The model under review builds one solid part; all positions refer to its coordinate system, in mm. Face numbers are marked on the shaded views. A direction names the side the tool comes from. Round coordinates to 2 decimals unless told otherwise and drop trailing zeros. Order: outer loops, then holes, each group sorted by start corner. A loop starts at its lowest first (then second) coordinate and runs counter-clockwise, first axis right, second up.
1) Consider section C-C (z = 13). Give the boundary of the cut face in (x, y), then the cut area to 3 significant figures.
2) Consider section A-A (y = -25.5). Give the boundary of the cut face in (x, z), then the cut area to 3 significant figures.
3) Clearance check with flat-ended pins moving along their axes: P1, Ø1.5, axis at x = 12.5, z = 12.5, coming from the -Y side; P2, Ø5, axis at x = -13, z = 13, coming from the -Y side; P3, Ø10.5, axis at x = -5, z = 8, coming from the -Y side. State where each tip first meets the part, or that it passes through.
4) Machinability: for the marked faces 1 and 2, which of the approach directions +Z, -Z, +X, -X, +Y, -Y give a long, thin tool a straight path to every point of the face, cutting with its end or side? Answer none if there is none.
5) To check wall thickness, follow L1, parallel to Z at x = -13, y = -13.5; L2, parallel to Z at x = 14, y = -8; L3, parallel to Y at x = 13.5, z = -4.5. State the ranges of each line that lie inside material, in increasing order.
6) Consider section D-D (z = -4). Give the boundary of the cut face in (x, y), then the cut area to 3 significant figures.
7) Consider section B-B (x = 13). Give the boundary of the cut face in (y, z), then the cut area to 3 significant figures.
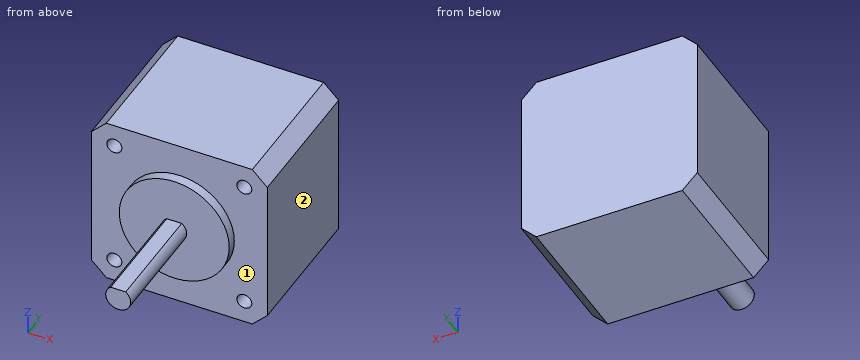
from build123d import *

# Parameters (mm, degrees)
F0_W     = 35.2
F0_H     = 35.2
F1_DEPTH = 28
F2_SIZE  = 3
F4_DEPTH = 24
F5_R     = 11
F6_DEPTH = 2
F7_R     = 1.5
F8_DEPTH = 25


with BuildPart() as f1:
    # F0 (on Front) → F1 (new body)
    with BuildSketch(Plane.XZ):
        Rectangle(F0_W, F0_H)
    extrude(amount=F1_DEPTH)

    # F2
    f2_edges = [f1.edges().sort_by_distance(p)[0] for p in [
        (-17.6, -14, 17.6),
        (-17.6, -14, -17.6),
        (17.6, -14, -17.6),
        (17.6, -14, 17.6),
    ]]
    chamfer(f2_edges, length=F2_SIZE)

    # F3 (on face) → F4 (join)
    with BuildSketch(Plane.XZ.offset(28)):
        with BuildLine():
            Line((1.5, 2), (-1.5, 2))
            ThreePointArc((-1.5, 2), (0, -2.5), (1.5, 2))
        make_face()
    extrude(amount=F4_DEPTH)

    # F5 (on face) → F6 (join)
    with BuildSketch(Plane.XZ.offset(28)):
        Circle(F5_R)
    extrude(amount=F6_DEPTH)

    # F7 (on face) → F8 (cut)
    with BuildSketch(Plane.XZ.offset(28)):
        with Locations((-13, 13)):
            Circle(F7_R)
        with Locations((13, 13)):
            Circle(F7_R)
        with Locations((13, -13)):
            Circle(F7_R)
        with Locations((-13, -13)):
            Circle(F7_R)
    extrude(amount=-F8_DEPTH, mode=Mode.SUBTRACT)


solid = f1.part
Answer below:
1. outline: (-17.6, -28) - (-14.5, -28) - (-14.5, -3) - (-11.5, -3) - (-11.5, -28) - (11.5, -28) - (11.5, -3) - (14.5, -3) - (14.5, -28) - (17.6, -28) - (17.6, 0) - (-17.6, 0) - close
1. area: 836 mm2
2. outline: (-17.6, -14.6) - (-14.6, -17.6) - (14.6, -17.6) - (17.6, -14.6) - (17.6, 14.6) - (14.6, 17.6) - (-14.6, 17.6) - (-17.6, 14.6) - close; hole circle Ø3 at (-13, -13); hole circle Ø3 at (-13, 13); hole circle Ø3 at (13, -13); hole circle Ø3 at (13, 13)
2. area: 1,190 mm2
3. P1: stops at y = -3
3. P2: stops at y = -28
3. P3: stops at y = -30
4. face 1: -Y
4. face 2: +Z, -Z, +X, +Y, -Y
5. L1: z = -17.6 to -14.5, -11.5 to 11.5, 14.5 to 17.6
5. L2: z = -17.6 to -14.12, -11.88 to 11.88, 14.12 to 17.6
5. L3: y = -28 to 0
6. outline: (-17.6, -28) - (-10.25, -28) - (-10.25, -30) - (10.25, -30) - (10.25, -28) - (17.6, -28) - (17.6, 0) - (-17.6, 0) - close
6. area: 1,030 mm2
7. outline: (-28, -17.6) - (0, -17.6) - (0, 17.6) - (-28, 17.6) - (-28, 14.5) - (-3, 14.5) - (-3, 11.5) - (-28, 11.5) - (-28, -11.5) - (-3, -11.5) - (-3, -14.5) - (-28, -14.5) - close
7. area: 836 mm2
